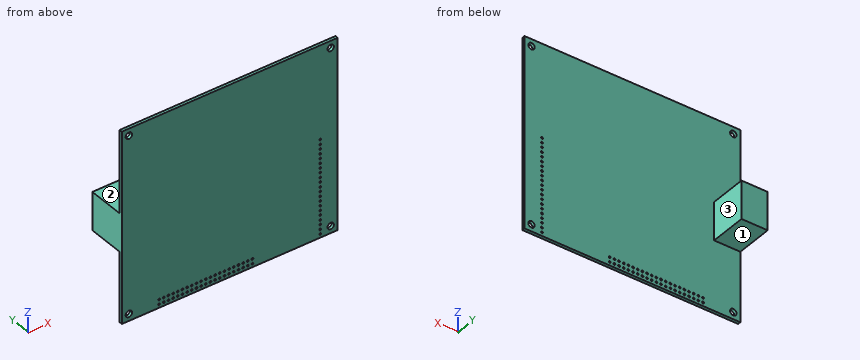
from build123d import *

# Parameters (mm, degrees)
SKETCH1_W           = 117.475
SKETCH1_H           = 103.505
SKETCH1_R           = 1.7526
BOSS_EXTRUDE1_DEPTH = 1.6
SKETCH2_W           = 14.25
SKETCH2_H           = 20.676
BOSS_EXTRUDE2_DEPTH = 20
SKETCH3_R           = 0.5
CUT_EXTRUDE1_DEPTH  = 2.6


with BuildPart() as part:
    # Sketch1 → Boss-Extrude1 (new body)
    with BuildSketch(Plane(origin=(0, 0, 0), x_dir=(1, 0, 0), z_dir=(0, 1, 0))):
        with Locations((58.7375, 51.7525)):
            Rectangle(SKETCH1_W, SKETCH1_H)
        with Locations((3.815, 3.815)):
            Circle(SKETCH1_R, mode=Mode.SUBTRACT)
        with Locations((113.66, 3.815)):
            Circle(SKETCH1_R, mode=Mode.SUBTRACT)
        with Locations((113.66, 99.69)):
            Circle(SKETCH1_R, mode=Mode.SUBTRACT)
        with Locations((3.815, 99.69)):
            Circle(SKETCH1_R, mode=Mode.SUBTRACT)
    extrude(amount=BOSS_EXTRUDE1_DEPTH)

    # Sketch2 → Boss-Extrude2 (add)
    with BuildSketch(Plane(origin=(0, 1.6, 0), x_dir=(1, 0, 0), z_dir=(0, 1, 0))):
        with Locations((7.125, 55.239)):
            Rectangle(SKETCH2_W, SKETCH2_H)
    extrude(amount=BOSS_EXTRUDE2_DEPTH)

    # Sketch3 → Cut-Extrude1 (cut, through all)
    with BuildSketch(Plane(origin=(0, 1.6, 0), x_dir=(1, 0, 0), z_dir=(0, 1, 0))):
        with Locations((20.285, 101.605)):
            Circle(SKETCH3_R)
        with Locations((22.825, 101.605)):
            Circle(SKETCH3_R)
        with Locations((25.365, 101.605)):
            Circle(SKETCH3_R)
        with Locations((27.905, 101.605)):
            Circle(SKETCH3_R)
        with Locations((30.445, 101.605)):
            Circle(SKETCH3_R)
        with Locations((32.985, 101.605)):
            Circle(SKETCH3_R)
        with Locations((35.525, 101.605)):
            Circle(SKETCH3_R)
        with Locations((38.065, 101.605)):
            Circle(SKETCH3_R)
        with Locations((40.605, 101.605)):
            Circle(SKETCH3_R)
        with Locations((43.145, 101.605)):
            Circle(SKETCH3_R)
        with Locations((45.685, 101.605)):
            Circle(SKETCH3_R)
        with Locations((48.225, 101.605)):
            Circle(SKETCH3_R)
        with Locations((50.765, 101.605)):
            Circle(SKETCH3_R)
        with Locations((53.305, 101.605)):
            Circle(SKETCH3_R)
        with Locations((55.845, 101.605)):
            Circle(SKETCH3_R)
        with Locations((58.385, 101.605)):
            Circle(SKETCH3_R)
        with Locations((60.925, 101.605)):
            Circle(SKETCH3_R)
        with Locations((63.465, 101.605)):
            Circle(SKETCH3_R)
        with Locations((66.005, 101.605)):
            Circle(SKETCH3_R)
        with Locations((68.545, 101.605)):
            Circle(SKETCH3_R)
        with Locations((71.085, 101.605)):
            Circle(SKETCH3_R)
        with Locations((22.825, 99.065)):
            Circle(SKETCH3_R)
        with Locations((25.365, 99.065)):
            Circle(SKETCH3_R)
        with Locations((27.905, 99.065)):
            Circle(SKETCH3_R)
        with Locations((30.445, 99.065)):
            Circle(SKETCH3_R)
        with Locations((32.985, 99.065)):
            Circle(SKETCH3_R)
        with Locations((35.525, 99.065)):
            Circle(SKETCH3_R)
        with Locations((38.065, 99.065)):
            Circle(SKETCH3_R)
        with Locations((40.605, 99.065)):
            Circle(SKETCH3_R)
        with Locations((43.145, 99.065)):
            Circle(SKETCH3_R)
        with Locations((45.685, 99.065)):
            Circle(SKETCH3_R)
        with Locations((48.225, 99.065)):
            Circle(SKETCH3_R)
        with Locations((50.765, 99.065)):
            Circle(SKETCH3_R)
        with Locations((53.305, 99.065)):
            Circle(SKETCH3_R)
        with Locations((55.845, 99.065)):
            Circle(SKETCH3_R)
        with Locations((58.385, 99.065)):
            Circle(SKETCH3_R)
        with Locations((60.925, 99.065)):
            Circle(SKETCH3_R)
        with Locations((63.465, 99.065)):
            Circle(SKETCH3_R)
        with Locations((66.005, 99.065)):
            Circle(SKETCH3_R)
        with Locations((68.545, 99.065)):
            Circle(SKETCH3_R)
        with Locations((71.085, 99.065)):
            Circle(SKETCH3_R)
        with Locations((20.285, 99.065)):
            Circle(SKETCH3_R)
        with Locations((107.97, 101.565)):
            Circle(SKETCH3_R)
        with Locations((107.97, 99.025)):
            Circle(SKETCH3_R)
        with Locations((107.97, 96.485)):
            Circle(SKETCH3_R)
        with Locations((107.97, 93.945)):
            Circle(SKETCH3_R)
        with Locations((107.97, 91.405)):
            Circle(SKETCH3_R)
        with Locations((107.97, 88.865)):
            Circle(SKETCH3_R)
        with Locations((107.97, 86.325)):
            Circle(SKETCH3_R)
        with Locations((107.97, 83.785)):
            Circle(SKETCH3_R)
        with Locations((107.97, 81.245)):
            Circle(SKETCH3_R)
        with Locations((107.97, 78.705)):
            Circle(SKETCH3_R)
        with Locations((107.97, 76.165)):
            Circle(SKETCH3_R)
        with Locations((107.97, 73.625)):
            Circle(SKETCH3_R)
        with Locations((107.97, 71.085)):
            Circle(SKETCH3_R)
        with Locations((107.97, 68.545)):
            Circle(SKETCH3_R)
        with Locations((107.97, 66.005)):
            Circle(SKETCH3_R)
        with Locations((107.97, 63.465)):
            Circle(SKETCH3_R)
        with Locations((107.97, 60.925)):
            Circle(SKETCH3_R)
        with Locations((107.97, 58.385)):
            Circle(SKETCH3_R)
        with Locations((107.97, 55.845)):
            Circle(SKETCH3_R)
        with Locations((107.97, 53.305)):
            Circle(SKETCH3_R)
        with Locations((107.97, 50.765)):
            Circle(SKETCH3_R)
    extrude(amount=-CUT_EXTRUDE1_DEPTH, mode=Mode.SUBTRACT)


solid = part.part
Here's how the part is built. I have some questions about the finished solid (model axes, mm). Face numbers are marked on the shaded views. A direction names the side the tool comes from. Give positions to 0.01 mm unless a question says otherwise; leave off trailing zeros. Order: outer loops, then holes, each group sorted by start corner. A loop starts at its lowest first (then second) coordinate and runs counter-clockwise, first axis right, second up. Notation, with made-up numbers: (20, 54) -> (31, 54) arc R18 cw to (31, 80) -> close; hole circle Ø1 at (65, -15). An arc over 180 degrees is marked (long way). Use a Markdown table: item, result. Add a question column.
Item 1: Imagine slicing it at D-D on x = 97. Please give me the cut outline in (y, z) (3 decimals), plus the area to 3 significant figures.
Item 2: Imagine slicing it at B-B on y = 11.5. Please give me the cut outline in (x, z).
Item 3: Imagine slicing it at C-C on z = -48.5. Please give me the cut outline in (x, y) (3 decimals).
Item 4: I need wall thicknesses on line 1 (Y direction, x = 37.5, z = -60.5); line 2 (X direction, y = 6.25, z = -62.5). Which ranges of each line are inside material? Lowest first, please.
Item 5: Imagine slicing it at A-A on x = 113.66. Please give me the cut outline in (y, z) (3 decimals).
Item 6: For the marked faces 1, 2 and 3, which set-ups out of +Z, -Z, +X, -X, +Y, -Y let a thin tool reach every point of the face, with its end or its side?
Item 7: Will these pins go through, and if not, where does the flat tip stop? pin 1 (5.5 mm diameter, centred on x = 113.66, z = -3.815, fed in from +Y); pin 2 (4.5 mm diameter, centred on x = 7, y = 7, fed in from -Z); pin 3 (7 mm diameter, centred on x = 6, y = 8, fed in from +Z).
Data:
| question | item | result |
|---|---|---|
| 1 | outline | (0, -103.505) -> (1.6, -103.505) -> (1.6, 0) -> (0, 0) -> close |
| 1 | area | 166 mm² |
| 2 | outline | (0, -65.58) -> (14.25, -65.58) -> (14.25, -44.9) -> (0, -44.9) -> close |
| 3 | outline | (0, 0) -> (117.475, 0) -> (117.475, 1.6) -> (14.25, 1.6) -> (14.25, 21.6) -> (0, 21.6) -> close |
| 4 | line 1 | y = 0 to 1.6 |
| 4 | line 2 | x = 0 to 14.25 |
| 5 | outline | (0, -103.505) -> (1.6, -103.505) -> (1.6, -101.443) -> (0, -101.443) -> close; (0, -97.937) -> (1.6, -97.937) -> (1.6, -5.568) -> (0, -5.568) -> close; (0, -2.062) -> (1.6, -2.062) -> (1.6, 0) -> (0, 0) -> close |
| 6 | face 1 | -Z, +X, -X, +Y |
| 6 | face 2 | +Z, +X, -X, +Y |
| 6 | face 3 | +Z, -Z, +X, +Y |
| 7 | pin 1 | stops at y = 1.6 |
| 7 | pin 2 | stops at z = -65.58 |
| 7 | pin 3 | stops at z = -44.9 |
